Autodesk Inventor part; units mm, degrees
ref_plane "YZ Plane" through (0, 0, 0) normal (1, 0, 0) x (0, 1, 0)
ref_plane "XZ Plane" through (0, 0, 0) normal (0, 1, 0) x (-1, 0, 0)
ref_plane "XY Plane" through (0, 0, 0) normal (0, 0, 1) x (1, 0, 0)
sketch "Sketch1" plane through (0, 0, 0) normal (0, 1, 0) x (-1, 0, 0)
  circle A0 centre (0, 0) radius 228.6
  line L0 (228.6, 0) -> (-228.6, 0) construction
  line L1 (0, -115.0592) -> (-99.6442, 57.5296) construction
  line L2 (-99.6442, 57.5296) -> (99.6442, 57.5296) construction
  line L3 (99.6442, 57.5296) -> (0, -115.0592) construction
  line L4 (99.6442, 57.5296) -> (74.2442, 57.5296) construction
  line L5 (99.6442, 57.5296) -> (86.9442, 35.5326) construction
  line L6 (-99.6442, 57.5296) -> (-74.2442, 57.5296) construction
  line L7 (-99.6442, 57.5296) -> (-86.9442, 35.5326) construction
  line L8 (0, -115.0592) -> (12.7, -93.0622) construction
  line L9 (0, -115.0592) -> (-12.7, -93.0622) construction
  dimension "d26" = 457.2
  dimension "d27" = 199.2884
  dimension "d28" = 25.4
  dimension "d29" = 25.4
  dimension "d30" = 25.4
  dimension "d31" = 25.4
  dimension "d32" = 25.4
  dimension "d33" = 25.4
extrude "Extrusion1" add sketch "Sketch1" along normal blind 6.35
hole "Hole1" at (-99.6442, 0, 57.5296) at (-74.2442, 0, 57.5296) at (-86.9442, 0, 35.5326) at (-12.7, 0, -93.0622) at (0, 0, -115.0592) at (12.7, 0, -93.0622) at (99.6442, 0, 57.5296) at (74.2442, 0, 57.5296) at (86.9442, 0, 35.5326) direction (0, 1, 0) diameter 3.9624 end through all
properties part number "Table"
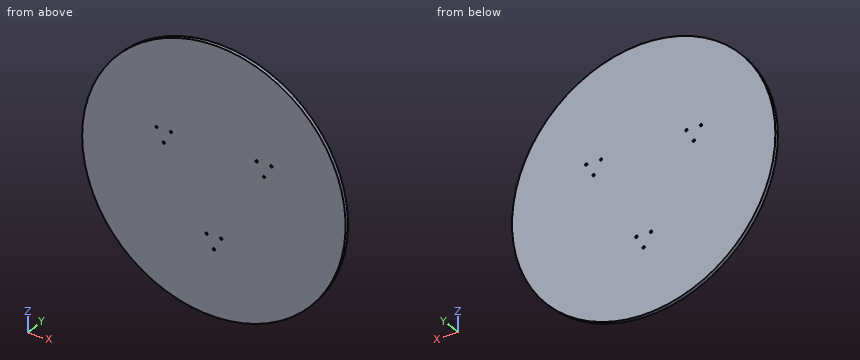
Here's how the part is built. I have some questions about the finished solid (model axes, mm). Round coordinates to 2 decimals unless told otherwise and drop trailing zeros. Order: outer loops, then holes, each group sorted by start corner. A loop starts at its lowest first (then second) coordinate and runs counter-clockwise, first axis right, second up. Notation, with made-up numbers: M 39,45 L 78,45 A14 ccw 78,59 Z; hole C -21,43 d7. An arc over 180 degrees is marked long. Answer in a Markdown table with one row per item.
Item 1: If I drill on L1, parallel to Z at x = 0, y = 3.75; L2, parallel to Z at x = -12.7, y = 2.5; L3, parallel to X at y = 4.5, z = 3.5, over which ranges is the centre line in solid material (lowest first)? Write a range as from..to.
A:
| item | result |
|---|---|
| L1 | z = -228.6..-117.04, -113.08..228.6 |
| L2 | z = -228.25..-95.04, -91.08..228.25 |
| L3 | x = -228.57..228.57 |
Item 2: Imagine slicing it at B-B, the plane x = -176.5. Write out the boundary of the cut face in (y, z).
A:
| item | result |
|---|---|
| outline | M 0,-145.28 L 6.35,-145.28 L 6.35,145.28 L 0,145.28 Z |
Item 3: Imagine slicing it at A-A, the plane y = 1.25. State how many separate pieces and enclosed holes the cut face has, and give its area (3 significant figures).
A:
| item | result |
|---|---|
| separate pieces | 1 |
| enclosed holes | 9 |
| area | 164,000 mm2 |
Item 4: Imagine slicing it at C-C, the plane z = -47. Write out the boundary of the cut face in (x, y), and give its area (3 significant figures).
A:
| item | result |
|---|---|
| outline | M -223.72,0 L 223.72,0 L 223.72,6.35 L -223.72,6.35 Z |
| area | 2,840 mm2 |
Item 5: I'm going to push flat-ended pins straight in: pin 1 (1.5 mm diameter, centred on y = 2, z = 8.5, fed in from +X); pin 2 (3 mm diameter, centred on y = 3, z = -49.5, fed in from +X); pin 3 (3.5 mm diameter, centred on x = 86.94, z = 35.53, fed in from -Y); pin 4 (1 mm diameter, centred on x = -41, y = 4.5, fed in from +Z). Where does each tip first touch, or does it pass through?
A:
| item | result |
|---|---|
| pin 1 | stops at x = 228.47 |
| pin 2 | stops at x = 223.5 |
| pin 3 | passes through |
| pin 4 | stops at z = 224.98 |
